Autodesk Inventor part; units mm, degrees
ref_plane "YZ Plane" through (0, 0, 0) normal (1, 0, 0) x (0, 1, 0)
ref_plane "XZ Plane" through (0, 0, 0) normal (0, 1, 0) x (-1, 0, 0)
ref_plane "XY Plane" through (0, 0, 0) normal (0, 0, 1) x (1, 0, 0)
sketch "Эскиз1" plane through (0, 0, 0) normal (0, 1, 0) x (-1, 0, 0)
  circle A0 centre (0, 0) radius 9.75
  dimension "d0" = 19.5
extrude "Выдавливание1" add sketch "Эскиз1" along normal blind 2
sketch "Эскиз5" plane through (0, 0, 0) normal (0, -1, 0) x (1, 0, 0)
  line L0 (5, -5) -> (-5, -5)
  line L1 (-5, -5) -> (-5, 5)
  line L2 (-5, 5) -> (5, 5)
  line L3 (5, 5) -> (5, -5)
  point P0 (0, 0)
  dimension "d12" = 10
  dimension "d13" = 10
  dimension "d17" = 5
  dimension "d27" = 5
extrude "Выдавливание5" add sketch "Эскиз5" along normal blind 5
sketch "Эскиз6" plane through (-5, 0, -5) normal (-1, 0, 0) x (0, 0, 1)
  circle A0 centre (5, -2.5) radius 1.35
  line L0 (10, -5) -> (0, -5)
  line L1 (0, 0) -> (0, -5)
  point P0 (5, 0)
  point P1 (0, -2.5)
  dimension "d30" = 2.7
  dimension "d31" = 2.5
  dimension "d32" = 5
extrude "Выдавливание6" cut sketch "Эскиз6" against normal blind 15.75
fillet "Сопряжение1" radius 5 4 edges at (5, -2.5, 5) (-5, -2.5, 5) (-5, -2.5, -5) (5, -2.5, -5)
sketch "Эскиз11" plane through (0, 2, 0) normal (0, 1, 0) x (1, 0, 0)
  circle A0 centre (0, 0) radius 5
  dimension "d47" = 10
extrude "Выдавливание9" add sketch "Эскиз11" along normal blind 3
sketch "Эскиз12" plane through (0, 5, 0) normal (0, 1, 0) x (1, 0, 0)
  circle A0 centre (0, 0) radius 9.75
  dimension "d50" = 19.5
extrude "Выдавливание10" add sketch "Эскиз12" along normal blind 2
sketch "Эскиз14" plane through (0, 7, 0) normal (0, 1, 0) x (1, 0, 0)
  circle A0 centre (0, 0) radius 2.5
  dimension "d56" = 5
extrude "Выдавливание12" add sketch "Эскиз14" along normal blind 1.5
sketch "Эскиз15" plane through (0, 8.5, 0) normal (0, 1, 0) x (1, 0, 0)
  circle A0 centre (0, 0) radius 2.15
  dimension "d59" = 4.3
extrude "Выдавливание13" cut sketch "Эскиз15" against normal blind 33.5
properties part number "koleso_left"
Can you work these out from the model? Positions are in its coordinate system, mm. A direction names the side the tool comes from. Coordinates: 2 decimals unless noted, no trailing zeros. Order: outer loops, then holes, each group sorted by start corner. A loop starts at its lowest first (then second) coordinate and runs counter-clockwise, first axis right, second up.
1. For faces 1 (the face through (-4, 0, -4)), 2 (the face through (-0.54, 7.74, -2.44)), 3 (the face through (-4, 2, -4)), which set-ups out of +Z, -Z, +X, -X, +Y, -Y let a thin tool reach every point of the face, with its end or its side?
2. I'm going to push flat-ended pins straight in: pin 1 (2 mm diameter, centred on x = 0.5, y = 3.5, fed in from +Z); pin 2 (6 mm diameter, centred on x = 6.5, y = 3.5, fed in from -Z); pin 3 (4 mm diameter, centred on x = -4.5, y = 2.5, fed in from -Z); pin 4 (1.6 mm diameter, centred on y = -2.5, z = 0, fed in from -X). Where does each tip first touch, or does it pass through?
3. If we section it at D-D (y = -2.5): Please give me the cut outline in (x, z).
4. If we section it at B-B (z = 0): Give the number of separate pieces and of enclosed holes in the cut face, then the cut area to 3 significant figures.
5. If we section it at C-C (z = -6): Please give me the cut outline in (x, y), then the cut area to 3 significant figures.
6. If we section it at A-A (x = 0): Please give me the cut outline in (y, z).
7. Thinking about a two-plate mould opening in Z: for faces 4 (the face through (2, 7, 2)), 5 (the face through (-1.08, 3.48, -4.88)), 6 (the face through (-3.36, -3.82, -0.29)), which applies, +Z half, -Z half, draft (parallel to the pull), parting line (faces both ways), or undercut?
8. I need wall thicknesses on line 1 (Y direction, x = -3.7, z = 0); line 2 (Y direction, x = -6, z = -2); line 3 (Z direction, x = 0, y = 2.5). Which ranges of each line are inside material? Lowest first, please.
Entries:
1. face 1: -Y
1. face 2: +Y
1. face 3: none
2. pin 1: stops at z = 5
2. pin 2: stops at z = -8.94
2. pin 3: stops at z = -9.41
2. pin 4: passes through
3. outline: (-4.81, -1.35) arc R5 ccw to (4.81, -1.35) - (1.67, -1.35) arc R2.15 cw to (-1.67, -1.35) - close; (-4.81, 1.35) - (-1.67, 1.35) arc R2.15 cw to (1.67, 1.35) - (4.81, 1.35) arc R5 ccw to start
4. separate pieces: 4
4. enclosed holes: 0
4. area: 92.1 mm2
5. outline: (-7.69, 0) - (7.69, 0) - (7.69, 2) - (-7.69, 2) - close; (-7.69, 5) - (7.69, 5) - (7.69, 7) - (-7.69, 7) - close
5. area: 61.5 mm2
6. outline: (-5, -5) - (0, -5) - (0, -9.75) - (2, -9.75) - (2, -5) - (5, -5) - (5, -9.75) - (7, -9.75) - (7, -2.5) - (8.5, -2.5) - (8.5, -2.15) - (-5, -2.15) - close; (-5, 2.15) - (8.5, 2.15) - (8.5, 2.5) - (7, 2.5) - (7, 9.75) - (5, 9.75) - (5, 5) - (2, 5) - (2, 9.75) - (0, 9.75) - (0, 5) - (-5, 5) - close
7. face 4: draft
7. face 5: parting line
7. face 6: undercut
8. line 1: y = -5 to -3.85, -1.15 to 7
8. line 2: y = 0 to 2, 5 to 7
8. line 3: z = -5 to -2.15, 2.15 to 5
